Read the model definition and answer for the solid it produces. Units are mm, in the model's axes. A direction names the side the tool comes from. Give positions to 0.01 mm unless a question says otherwise; leave off trailing zeros. Write each loop counter-clockwise with the first axis right and the second up, starting at its lowest first coordinate (ties: lowest second). Pieces come first, ordered by that corner, then holes. Notation, with made-up numbers: (7, 70) -> (35, 70) arc R26 ccw to (35, 92) -> close; hole circle Ø7 at (45, 33). An arc over 180 degrees is marked (long way). Write item = value, one per line.
from build123d import *

# Parameters (mm, degrees)
F0_W     = 82.55
F0_H     = 77.089
F1_DEPTH = 25.4
F2_W     = 82.55
F2_H     = 77.089
F3_DEPTH = 3.6195
F4_R     = 5.08
F5_R     = 5.08


with BuildPart() as f1:
    # F0 (on Top) → F1 (new body)
    with BuildSketch(Plane.XY):
        Polygon((-44.8945, 42.164), (-44.8945, 38.5445), (-44.8945, -42.164), (44.8945, -42.164), (44.8945, 42.164), align=None)
        Rectangle(F0_W, F0_H, mode=Mode.SUBTRACT)
    extrude(amount=F1_DEPTH)

    # F2 (on face) → F3 (join)
    with BuildSketch(Plane.XY.offset(25.4)):
        Rectangle(F2_W, F2_H)
    extrude(amount=-F3_DEPTH)

    # F4
    f4_edges = [f1.edges().sort_by_distance(p)[0] for p in [
        (41.275, -38.5445, 10.89025),
        (-41.275, -38.5445, 10.89025),
        (41.275, 38.5445, 10.89025),
        (-41.275, 38.5445, 10.89025),
    ]]
    fillet(f4_edges, radius=F4_R)

    # F5
    f5_edges = [f1.edges().sort_by_distance(p)[0] for p in [
        (-44.8945, -42.164, 12.7),
        (44.8945, -42.164, 12.7),
        (44.8945, 42.164, 12.7),
        (-44.8945, 42.164, 12.7),
        (0, 42.164, 25.4),
        (-44.8945, 0, 25.4),
        (0, -42.164, 25.4),
        (44.8945, 0, 25.4),
    ]]
    fillet(f5_edges, radius=F5_R)


solid = f1.part
(1) The part is cut by section C-C on x = -33. Determine the outline of the cut face in (y, z), plus the area to 3 significant figures.
Checks:
outline = (-42.16, 0) -> (-38.54, 0) -> (-38.54, 21.78) -> (38.54, 21.78) -> (38.54, 0) -> (42.16, 0) -> (42.16, 20.32) arc R5.08 ccw to (37.08, 25.4) -> (-37.08, 25.4) arc R5.08 ccw to (-42.16, 20.32) -> close
area = 452 mm²
(2) The part is cut by section B-B on z = 18.5. Determine the outline of the cut face in (x, y) (1 decimal), plus the area to 3 significant figures.
Checks:
outline = (-44.9, -37.1) arc R5.1 ccw to (-39.8, -42.2) -> (39.8, -42.2) arc R5.1 ccw to (44.9, -37.1) -> (44.9, 37.1) arc R5.1 ccw to (39.8, 42.2) -> (-39.8, 42.2) arc R5.1 ccw to (-44.9, 37.1) -> close; hole (-41.3, -33.5) arc R5.1 ccw to (-36.2, -38.5) -> (36.2, -38.5) arc R5.1 ccw to (41.3, -33.5) -> (41.3, 33.5) arc R5.1 ccw to (36.2, 38.5) -> (-36.2, 38.5) arc R5.1 ccw to (-41.3, 33.5) -> close
area = 1,210 mm²
(3) For a pull along X with two mould halves and no side action, classify faces 1 (the flat face through (-1, 1, 25.4)), 2 (the cylindrical face through (-39.747, -37.096, 11.043)), 3 (the cylindrical face through (-43.446, 40.636, 10.302)) as released by +X, released by -X, zero draft, split by the parting line, or undercut.
Checks:
face_1 = zero draft
face_2 = undercut
face_3 = released by -X
(4) The part is cut by section A-A on y = -9. Determine the outline of the cut face in (x, z) (1 decimal), plus the area to 3 significant figures.
Checks:
outline = (-44.9, 0) -> (-41.3, 0) -> (-41.3, 21.8) -> (41.3, 21.8) -> (41.3, 0) -> (44.9, 0) -> (44.9, 20.3) arc R5.1 ccw to (39.8, 25.4) -> (-39.8, 25.4) arc R5.1 ccw to (-44.9, 20.3) -> close
area = 472 mm²
(5) Given P1, Ø3, axis at y = 25.5, z = 22, coming from the +X side, flat-ended and moving along its own axis, determine where the tip first touches the part or whether it passes through.
Checks:
P1 = 44.89
(6) Consider L1, parallel to Y at x = 15, z = 16.25; L2, parallel to X at y = -10.5, z = 14.25 (1 decimal); L3, parallel to Z at x = 18.5, y = 23. Determine where each line is inside the solid, lowest interval first.
Checks:
L1 = -42.16 to -38.54, 38.54 to 42.16
L2 = -44.9 to -41.3, 41.3 to 44.9
L3 = 21.78 to 25.4
(7) A tool of negligible diameter and unlimited length cuts with its end or side. For faces 4 (the flat face through (1, 42.164, 10)), 5 (the cylindrical face through (39.826, 37.017, 11.043)), from which of +Z, -Z, +X, -X, +Y, -Y can it reach the whole face along a straight path? Write none if from no direction.
Checks:
face_4 = +Z, -Z, +X, -X, +Y
face_5 = -Z
